The listing builds one solid part. Answer for the finished solid, in the listing's coordinates (mm). Round coordinates to 2 decimals unless told otherwise and drop trailing zeros. Write each loop counter-clockwise with the first axis right and the second up, starting at its lowest first coordinate (ties: lowest second). Pieces come first, ordered by that corner, then holes. Notation, with made-up numbers: M 23.5,-26.75 L 29.5,-26.75 A20 cw 29.5,-7.75 Z; hole C 44,47.5 d3. An arc over 180 degrees is marked long. One line per item, written item: value. Start each with the question number.
(1) Consider probe 1 along Z at (x, y) = (3, -4.5); probe 2 along Y at (x, z) = (-0.5, 2.25); probe 3 along Y at (x, z) = (5, 7.5) (3 decimals). Determine where each line is inside the solid, lowest interval first.
(2) Given P1, Ø1, axis at x = 5, z = 12.5, coming from the -Y side; P2, Ø5, axis at y = -4.5, z = 4.5, coming from the -X side; P3, Ø2, axis at y = -4.5, z = 3, coming from the +X side, each flat-ended and moving along its own axis, determine where each tip first touches the part or whether it passes through.
(3) Section A-A (z = 3.25) is taken. Determine the outline of the cut face in (x, y).
```python
from build123d import *

# Parameters (mm, degrees)
SKETCH2_R           = 8
BOSS_EXTRUDE1_DEPTH = 17
CHAMFER1_SIZE       = 1
CHAMFER1_SIZE2      = 1.732050808
SKETCH5_R           = 6.064278786
CUT_EXTRUDE1_DEPTH  = 0.1
SKETCH6_R           = 5
BOSS_EXTRUDE4_DEPTH = 0.1


with BuildPart() as part:
    # Sketch2 → Boss-Extrude1 (new body)
    with BuildSketch(Plane.XY):
        Circle(SKETCH2_R)
    extrude(amount=BOSS_EXTRUDE1_DEPTH)

    # Chamfer1
    chamfer1_edges = [part.edges().sort_by_distance(p)[0] for p in [
        (-8, 0, 17),
    ]]
    chamfer1_side = [part.faces().sort_by_distance(p)[0] for p in [
        (-8, 0, 8.5),
    ]]
    chamfer(chamfer1_edges, length=CHAMFER1_SIZE, length2=CHAMFER1_SIZE2, reference=chamfer1_side[0])

    # Sketch5 → Cut-Extrude1 (cut)
    with BuildSketch(Plane.XY.offset(17)):
        Circle(SKETCH5_R)
    extrude(amount=-CUT_EXTRUDE1_DEPTH, mode=Mode.SUBTRACT)

    # Sketch6 → Boss-Extrude4 (add)
    with BuildSketch(Plane.XY.offset(16.9)):
        Circle(SKETCH6_R)
    extrude(amount=BOSS_EXTRUDE4_DEPTH)


solid = part.part
```
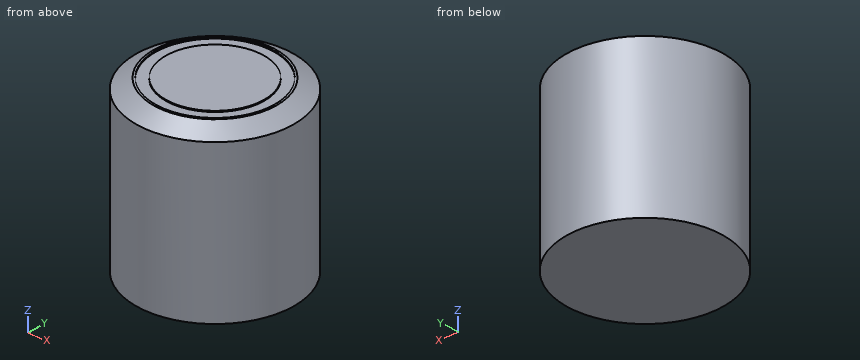
Recorded:
1. probe 1: z = 0 to 16.9
1. probe 2: y = -7.98 to 7.98
1. probe 3: y = -6.245 to 6.245
2. P1: stops at y = -6.61
2. P2: stops at x = -7.75
2. P3: stops at x = 7.19
3. outline: C 0,0 d16
